Can you work these out from the model? Positions are in its coordinate system, mm. A direction names the side the tool comes from. Give positions to 0.01 mm unless a question says otherwise; leave off trailing zeros. Loops run counter-clockwise (first coordinate to the right, second up) from the corner with the lowest first, then second, coordinate; pieces in that order, holes last. Notation, with made-up numbers: (10.25, 4.5) -> (29.25, 4.5) arc R27 ccw to (29.25, 24.5) -> close; hole circle Ø10 at (-15, -3). An arc over 180 degrees is marked (long way). Return JSON: item names as keys, results as strings. Group by question number.
Q1. Suppose I cut it at D-D, the plane y = 1. Count the separate pieces of the cut face and the enclosed holes in it, and give its area (3 significant figures).
Q2. Which directions (+Z, -Z, +X, -X, +Y, -Y) give clear straight access to the entire face, cutting with the end or side of a thin tool? Please do faces 5 (the cylindrical face through (-23.784, 1.972, -26.115)), 6 (the flat face through (21, 2, -23)), 7 (the flat face through (25, 4, 23)), 8 (the flat face through (21, 2, 24)).
Q3. I need wall thicknesses on line 1 along X through (y, z) = (1.1, 25); line 2 along Z through (x, y) = (-25, 1.4); line 3 along Z through (x, y) = (-21, 12.25). Which ranges of each line are inside material? Lowest first, please. Write a range as [from, to].
Q4. Will these pins go through, and if not, where does the flat tip stop? pin 1 (4 mm diameter, centred on x = -15.5, z = -5.5, fed in from -Y); pin 2 (8 mm diameter, centred on x = 13.5, y = 12, fed in from +Z); pin 3 (12 mm diameter, centred on x = 18.5, z = 5.5, fed in from +Y); pin 4 (3 mm diameter, centred on x = -9.5, y = 9, fed in from -Z).
Q5. Thinking about a two-plate mould opening in X: for faces 1 (the flat face through (0, 8, 21)), 2 (the flat face through (25, 4, -23)), 3 (the cylindrical face through (-23.784, 1.972, 23.885)), 4 (the flat face through (-32, 3.8, 4.7)), which applies, pulls with the +X half, pulls with the -X half, needs draft (parallel to the pull), parting line crosses it, or undercut?
Q6. Suppose I cut it at A-A, the plane y = 10.25. Please give me the cut outline in (x, z).
Q7. Suppose I cut it at B-B, the plane x = -25. Please give me the cut outline in (y, z), and give its area (3 significant figures).
Q8. Suppose I cut it at C-C, the plane x = -8. Please give me the cut outline in (y, z), and give its area (3 significant figures).
```python
from build123d import *

# Parameters (mm, degrees)
BOSS_EXTRUDE1_DEPTH   = 14
CUT_EXTRUDE1_START    = -10
CUT_EXTRUDE1_DEPTH    = 10
M4X0_7_TAPPED_HOLE1_D = 3.3
FILLET2_R             = 1


with BuildPart() as part:
    # Sketch1 → Boss-Extrude1 (new body)
    with BuildSketch(Plane(origin=(0, 0, 0), x_dir=(1, 0, 0), z_dir=(0, 1, 0))):
        with BuildLine():
            Line((-31, 21), (-30, 21))
            ThreePointArc((-30, 21), (-29.292893219, 21.292893219), (-29, 22))
            Line((-29, 22), (-29, 25))
            ThreePointArc((-29, 25), (-25, 29), (-21, 25))
            Line((-21, 25), (-21, 22))
            ThreePointArc((-21, 22), (-20.707106781, 21.292893219), (-20, 21))
            Line((-20, 21), (20, 21))
            ThreePointArc((20, 21), (20.707106781, 21.292893219), (21, 22))
            Line((21, 22), (21, 25))
            ThreePointArc((21, 25), (25, 29), (29, 25))
            Line((29, 25), (29, 22))
            ThreePointArc((29, 22), (29.292893219, 21.292893219), (30, 21))
            Line((30, 21), (31, 21))
            ThreePointArc((31, 21), (31.707106781, 20.707106781), (32, 20))
            Line((32, 20), (32, -20))
            ThreePointArc((32, -20), (31.707106781, -20.707106781), (31, -21))
            Line((31, -21), (30, -21))
            ThreePointArc((30, -21), (29.292893219, -21.292893219), (29, -22))
            Line((29, -22), (29, -25))
            ThreePointArc((29, -25), (25, -29), (21, -25))
            Line((21, -25), (21, -22))
            ThreePointArc((21, -22), (20.707106781, -21.292893219), (20, -21))
            Line((20, -21), (-20, -21))
            ThreePointArc((-20, -21), (-20.707106781, -21.292893219), (-21, -22))
            Line((-21, -22), (-21, -25))
            ThreePointArc((-21, -25), (-25, -29), (-29, -25))
            Line((-29, -25), (-29, -22))
            ThreePointArc((-29, -22), (-29.292893219, -21.292893219), (-30, -21))
            Line((-30, -21), (-31, -21))
            ThreePointArc((-31, -21), (-31.707106781, -20.707106781), (-32, -20))
            Line((-32, -20), (-32, 20))
            ThreePointArc((-32, 20), (-31.707106781, 20.707106781), (-31, 21))
        make_face()
    extrude(amount=BOSS_EXTRUDE1_DEPTH)

    # Sketch2 → Cut-Extrude1 (cut)
    with BuildSketch(Plane(origin=(0, 14, 0), x_dir=(1, 0, 0), z_dir=(0, 1, 0)).offset(CUT_EXTRUDE1_START)):
        with BuildLine():
            Line((-30, -21), (-20, -21))
            ThreePointArc((-20, -21), (-20.707106781, -21.292893219), (-21, -22))
            Line((-21, -22), (-21, -25))
            ThreePointArc((-21, -25), (-25, -29), (-29, -25))
            Line((-29, -25), (-29, -22))
            ThreePointArc((-29, -22), (-29.292893219, -21.292893219), (-30, -21))
        make_face()
        Polygon((-29.25, 18.5), (29.25, 18.5), (29.25, 17), (32, 17), (32, -17), (29.25, -17), (29.25, -18.5), (-29.25, -18.5), (-29.25, -17), (-32, -17), (-32, 17), (-29.25, 17), align=None)
        with BuildLine():
            Line((21, -25), (21, -22))
            ThreePointArc((21, -22), (20.707106781, -21.292893219), (20, -21))
            Line((20, -21), (30, -21))
            ThreePointArc((30, -21), (29.292893219, -21.292893219), (29, -22))
            Line((29, -22), (29, -25))
            ThreePointArc((29, -25), (25, -29), (21, -25))
        make_face()
        with BuildLine():
            Line((30, 21), (20, 21))
            ThreePointArc((20, 21), (20.707106781, 21.292893219), (21, 22))
            Line((21, 22), (21, 25))
            ThreePointArc((21, 25), (25, 29), (29, 25))
            Line((29, 25), (29, 22))
            ThreePointArc((29, 22), (29.292893219, 21.292893219), (30, 21))
        make_face()
        with BuildLine():
            Line((-21, 25), (-21, 22))
            ThreePointArc((-21, 22), (-20.707106781, 21.292893219), (-20, 21))
            Line((-20, 21), (-30, 21))
            ThreePointArc((-30, 21), (-29.292893219, 21.292893219), (-29, 22))
            Line((-29, 22), (-29, 25))
            ThreePointArc((-29, 25), (-25, 29), (-21, 25))
        make_face()
    extrude(amount=CUT_EXTRUDE1_DEPTH, mode=Mode.SUBTRACT)

    # M4x0.7 Tapped Hole1 (through all)
    with Locations(Plane(origin=(0, 4, 0), x_dir=(1, 0, 0), z_dir=(0, 1, 0))):
        with Locations((-25, 25), (25, 25), (25, -25), (-25, -25)):
            Hole(M4X0_7_TAPPED_HOLE1_D / 2)

    # Fillet2
    fillet2_edges = [part.edges().sort_by_distance(p)[0] for p in [
        (-29.25, 9, -17),
        (29.25, 9, -17),
        (32, 9, -17),
        (32, 9, 17),
        (29.25, 9, 17),
        (-29.25, 9, 17),
        (-32, 9, 17),
        (-32, 9, -17),
    ]]
    fillet(fillet2_edges, radius=FILLET2_R)


solid = part.part
```
Ans:
{
 "1": {"separate pieces": "1", "enclosed holes": "4", "area": "2,880 mm^2"},
 "2": {"face 5": "+Y, -Y", "face 6": "-Z, +Y, -Y", "face 7": "+Z, +X, -X, +Y", "face 8": "+Z, +Y, -Y"},
 "3": {"line 1": "x = [-29, -26.65], [-23.35, -21], [21, 23.35], [26.65, 29]", "line 2": "z = [-29, -26.65], [-23.35, 23.35], [26.65, 29]", "line 3": "z = [-21, -18.5], [18.5, 21]"},
 "4": {"pin 1": "stops at y = 0", "pin 2": "stops at z = 21", "pin 3": "stops at y = 4", "pin 4": "stops at z = -21"},
 "5": {"face 1": "undercut", "face 2": "needs draft", "face 3": "undercut", "face 4": "pulls with the -X half"},
 "6": {"outline": "(-32, -20) arc R1 ccw to (-31, -21) -> (31, -21) arc R1 ccw to (32, -20) -> (32, -18) arc R1 ccw to (31, -17) -> (30.25, -17) arc R1 ccw to (29.25, -18) -> (29.25, -18.5) -> (-29.25, -18.5) -> (-29.25, -18) arc R1 ccw to (-30.25, -17) -> (-31, -17) arc R1 ccw to (-32, -18) -> close; (-32, 18) arc R1 ccw to (-31, 17) -> (-30.25, 17) arc R1 ccw to (-29.25, 18) -> (-29.25, 18.5) -> (29.25, 18.5) -> (29.25, 18) arc R1 ccw to (30.25, 17) -> (31, 17) arc R1 ccw to (32, 18) -> (32, 20) arc R1 ccw to (31, 21) -> (-31, 21) arc R1 ccw to (-32, 20) -> close"},
 "7": {"outline": "(0, -29) -> (4, -29) -> (4, -26.65) -> (0, -26.65) -> close; (0, -23.35) -> (4, -23.35) -> (4, -21) -> (14, -21) -> (14, -18.5) -> (4, -18.5) -> (4, 18.5) -> (14, 18.5) -> (14, 21) -> (4, 21) -> (4, 23.35) -> (0, 23.35) -> close; (0, 26.65) -> (4, 26.65) -> (4, 29) -> (0, 29) -> close", "area": "256 mm^2"},
 "8": {"outline": "(0, -21) -> (14, -21) -> (14, -18.5) -> (4, -18.5) -> (4, 18.5) -> (14, 18.5) -> (14, 21) -> (0, 21) -> close", "area": "218 mm^2"}
}
